from build123d import *

# Parameters (mm, degrees)
SKETCH5_W           = 2.54
SKETCH5_H           = 1.778
BOSS_EXTRUDE3_DEPTH = 58.166
SKETCH6_R           = 0.635
CUT_EXTRUDE3_DEPTH  = 3.54
SKETCH8_R           = 0.635
CUT_EXTRUDE4_DEPTH  = 3.54


with BuildPart() as part:
    # Sketch5 → Boss-Extrude3 (new body)
    with BuildSketch(Plane(origin=(0, 0, 0), x_dir=(0, 0, -1), z_dir=(1, 0, 0))):
        with Locations((1.27, 0.889)):
            Rectangle(SKETCH5_W, SKETCH5_H)
    extrude(amount=BOSS_EXTRUDE3_DEPTH)

    # Sketch6 → Cut-Extrude3 (cut, through all)
    with BuildSketch(Plane.XY):
        with Locations((5.5372, 0.889)):
            Circle(SKETCH6_R)
    extrude(amount=-CUT_EXTRUDE3_DEPTH, mode=Mode.SUBTRACT)

    # Sketch8 → Cut-Extrude4 (cut, through all)
    with BuildSketch(Plane.XY):
        with Locations((41.4782, 0.889)):
            Circle(SKETCH8_R)
        with Locations((51.2572, 0.889)):
            Circle(SKETCH8_R)
    extrude(amount=-CUT_EXTRUDE4_DEPTH, mode=Mode.SUBTRACT)


solid = part.part
CAD build for the part. Positions are in the model's coordinates, mm. Round coordinates to 2 decimals unless told otherwise and drop trailing zeros. Order: outer loops, then holes, each group sorted by start corner. A loop starts at its lowest first (then second) coordinate and runs counter-clockwise, first axis right, second up. Notation, with made-up numbers: M 52,84.25 L 84,84.25 A12 cw 84,98.25 Z; hole C 51,56 d11. An arc over 180 degrees is marked long. Use one line per item in the form item = value.
Q1. Two-plate mould, pull along X, no slides. Class faces 1 (the flat face through (29, 1, 0)), 2 (the cylindrical face through (51.863, 1.08, -1.252)), 3 (the flat face through (58.166, 1, -1)): +X half, -X half, draft (parallel to the pull), parting line (faces both ways), or undercut.
Recorded:
face_1 = draft
face_2 = undercut
face_3 = +X half
Q2. Probe L1, parallel to X at y = 0.85, z = -1.05; L2, parallel to X at y = 1.1, z = -0.5. List the from-to ranges inside material, lowest first.
Recorded:
L1 = 0 to 4.9, 6.17 to 40.84, 42.11 to 50.62, 51.89 to 58.17
L2 = 0 to 4.94, 6.14 to 40.88, 42.08 to 50.66, 51.86 to 58.17
Q3. Saw through at A-A on y = 0.55. Give the cut face in (x, z).
Recorded:
outline = M 0,-2.54 L 5,-2.54 L 5,0 L 0,0 Z; M 6.07,-2.54 L 40.94,-2.54 L 40.94,0 L 6.07,0 Z; M 42.02,-2.54 L 50.72,-2.54 L 50.72,0 L 42.02,0 Z; M 51.79,-2.54 L 58.17,-2.54 L 58.17,0 L 51.79,0 Z
Q4. Saw through at B-B on z = -1.75. Give the cut face in (x, y) (3 decimals), then the cut area to 3 significant figures.
Recorded:
outline = M 0,0 L 58.166,0 L 58.166,1.778 L 0,1.778 Z; hole C 5.537,0.889 d1.27; hole C 41.478,0.889 d1.27; hole C 51.257,0.889 d1.27
area = 99.6 mm^2
Q5. Flat gauge pin, fed straight in: P1, Ø1, axis at x = 17, y = 0.5, coming from the +Z side. Where does the tip first touch, or does it go through?
Recorded:
P1 = 0
